The model under review builds one solid part; all positions refer to its coordinate system, in mm. Coordinates: 2 decimals unless noted, no trailing zeros. Use one line per item in the form item = value.
from build123d import *

# Parameters (mm, degrees)
SKETCH1_R           = 5.25
BOSS_EXTRUDE1_DEPTH = 500


with BuildPart() as part:
    # Sketch1 → Boss-Extrude1 (new body)
    with BuildSketch(Plane(origin=(0, 0, -200), x_dir=(-1, 0, 0), z_dir=(0, 0, -1))):
        with BuildLine():
            Line((19.5, 22.5), (5, 22.5))
            Line((5, 22.5), (5, 16.5))
            Line((5, 16.5), (10, 16.5))
            Line((10, 16.5), (10, 12.121320344))
            Line((10, 12.121320344), (7.378679656, 9.5))
            Line((7.378679656, 9.5), (3.346410162, 9.5))
            Line((3.346410162, 9.5), (3, 9.3))
            Line((3, 9.3), (2.653589838, 9.5))
            Line((2.653589838, 9.5), (0.519615242, 9.5))
            Line((0.519615242, 9.5), (0, 9.2))
            Line((0, 9.2), (-0.519615242, 9.5))
            Line((-0.519615242, 9.5), (-2.653589838, 9.5))
            Line((-2.653589838, 9.5), (-3, 9.3))
            Line((-3, 9.3), (-3.346410162, 9.5))
            Line((-3.346410162, 9.5), (-7.378679656, 9.5))
            Line((-7.378679656, 9.5), (-10, 12.121320344))
            Line((-10, 12.121320344), (-10, 16.5))
            Line((-10, 16.5), (-5, 16.5))
            Line((-5, 16.5), (-5, 22.5))
            Line((-5, 22.5), (-19.5, 22.5))
            ThreePointArc((-19.5, 22.5), (-21.621320344, 21.621320344), (-22.5, 19.5))
            Line((-22.5, 19.5), (-22.5, 5))
            Line((-22.5, 5), (-16.5, 5))
            Line((-16.5, 5), (-16.5, 10))
            Line((-16.5, 10), (-12.121320344, 10))
            Line((-12.121320344, 10), (-9.5, 7.378679656))
            Line((-9.5, 7.378679656), (-9.5, 3.346410162))
            Line((-9.5, 3.346410162), (-9.3, 3))
            Line((-9.3, 3), (-9.5, 2.653589838))
            Line((-9.5, 2.653589838), (-9.5, 0.519615242))
            Line((-9.5, 0.519615242), (-9.2, 0))
            Line((-9.2, 0), (-9.5, -0.519615242))
            Line((-9.5, -0.519615242), (-9.5, -2.653589838))
            Line((-9.5, -2.653589838), (-9.3, -3))
            Line((-9.3, -3), (-9.5, -3.346410162))
            Line((-9.5, -3.346410162), (-9.5, -7.378679656))
            Line((-9.5, -7.378679656), (-12.121320344, -10))
            Line((-12.121320344, -10), (-16.5, -10))
            Line((-16.5, -10), (-16.5, -5))
            Line((-16.5, -5), (-22.5, -5))
            Line((-22.5, -5), (-22.5, -19.5))
            ThreePointArc((-22.5, -19.5), (-21.621320344, -21.621320344), (-19.5, -22.5))
            Line((-19.5, -22.5), (-5, -22.5))
            Line((-5, -22.5), (-5, -16.5))
            Line((-5, -16.5), (-10, -16.5))
            Line((-10, -16.5), (-10, -12.121320344))
            Line((-10, -12.121320344), (-7.378679656, -9.5))
            Line((-7.378679656, -9.5), (-3.346410162, -9.5))
            Line((-3.346410162, -9.5), (-3, -9.3))
            Line((-3, -9.3), (-2.653589838, -9.5))
            Line((-2.653589838, -9.5), (-0.519615242, -9.5))
            Line((-0.519615242, -9.5), (0, -9.2))
            Line((0, -9.2), (0.519615242, -9.5))
            Line((0.519615242, -9.5), (2.653589838, -9.5))
            Line((2.653589838, -9.5), (3, -9.3))
            Line((3, -9.3), (3.346410162, -9.5))
            Line((3.346410162, -9.5), (7.378679656, -9.5))
            Line((7.378679656, -9.5), (10, -12.121320344))
            Line((10, -12.121320344), (10, -16.5))
            Line((10, -16.5), (5, -16.5))
            Line((5, -16.5), (5, -22.5))
            Line((5, -22.5), (19.5, -22.5))
            ThreePointArc((19.5, -22.5), (21.621320344, -21.621320344), (22.5, -19.5))
            Line((22.5, -19.5), (22.5, -5))
            Line((22.5, -5), (16.5, -5))
            Line((16.5, -5), (16.5, -10))
            Line((16.5, -10), (12.121320344, -10))
            Line((12.121320344, -10), (9.5, -7.378679656))
            Line((9.5, -7.378679656), (9.5, -3.346410162))
            Line((9.5, -3.346410162), (9.3, -3))
            Line((9.3, -3), (9.5, -2.653589838))
            Line((9.5, -2.653589838), (9.5, -0.519615242))
            Line((9.5, -0.519615242), (9.2, 0))
            Line((9.2, 0), (9.5, 0.519615242))
            Line((9.5, 0.519615242), (9.5, 2.653589838))
            Line((9.5, 2.653589838), (9.3, 3))
            Line((9.3, 3), (9.5, 3.346410162))
            Line((9.5, 3.346410162), (9.5, 7.378679656))
            Line((9.5, 7.378679656), (12.121320344, 10))
            Line((12.121320344, 10), (16.5, 10))
            Line((16.5, 10), (16.5, 5))
            Line((16.5, 5), (22.5, 5))
            Line((22.5, 5), (22.5, 19.5))
            ThreePointArc((22.5, 19.5), (21.621320344, 21.621320344), (19.5, 22.5))
        make_face()
        with Locations(Location((0, 0, 0), (0, 0, 180))):
            Circle(SKETCH1_R, mode=Mode.SUBTRACT)
    extrude(amount=-BOSS_EXTRUDE1_DEPTH)


solid = part.part
Item 1: Draft analysis for pull direction Y (two halves, no side actions). For faces 1 (the face through (12, -22.5, 46)), 2 (the face through (5, -1.6, 46.5)), 3 (the face through (5, 5, 300)), state which applies: released by +Y, released by -Y, zero draft, split by the parting line, or undercut.
Results found:
face_1 = released by -Y
face_2 = undercut
face_3 = zero draft
Item 2: To check wall thickness, follow L1, parallel to X at y = -1, z = 33.5; L2, parallel to Y at x = 0, z = 170; L3, parallel to Y at x = -18.5, z = -3. State the ranges of each line that lie inside material, in increasing order. Write a range as from..to.
Results found:
L1 = -9.5..-5.15, 5.15..9.5
L2 = -9.2..-5.25, 5.25..9.2
L3 = -22.5..-5, 5..22.5
Item 3: Clearance check with flat-ended pins moving along their axes: pin 1 (4 mm diameter, centred on y = -2.5, z = 90.5, fed in from +X); pin 2 (2.5 mm diameter, centred on x = 2, z = -30, fed in from -Y); pin 3 (0.6 mm diameter, centred on x = 1, z = -25, fed in from +Y); pin 4 (6.5 mm diameter, centred on x = 0, y = 0, fed in from +Z). State where each tip first meets the part, or that it passes through.
Results found:
pin_1 = 9.5
pin_2 = -9.5
pin_3 = 9.5
pin_4 = through
